```python
from build123d import *

# Parameters (mm, degrees)
SKETCH1_W           = 89.6
SKETCH1_H           = 100.6
BOSS_EXTRUDE1_DEPTH = 49.7
SKETCH4_W           = 16.6
SKETCH4_H           = 12
CUT_EXTRUDE1_DEPTH  = 120.117546986
SKETCH5_W           = 100.6
SKETCH5_H           = 3
BOSS_EXTRUDE2_DEPTH = 89.6
SKETCH7_R           = 4.175
BOSS_EXTRUDE3_DEPTH = 21.7
CUT_EXTRUDE2_START  = 21.7
SKETCH7_3_R         = 2.175
CUT_EXTRUDE2_DEPTH  = 5
SKETCH9_R           = 4.675
SKETCH9_R_2         = 2.175
BOSS_EXTRUDE4_DEPTH = 3.5
CUT_EXTRUDE4_START  = -1.5
SKETCH9_2_R         = 2.175
CUT_EXTRUDE4_DEPTH  = 1.5
SKETCH11_W          = 21.5
SKETCH11_H          = 17.55
SKETCH11_W_2        = 4.5
SKETCH11_H_2        = 7.5
BOSS_EXTRUDE5_DEPTH = 3.5
SKETCH12_W          = 17
SKETCH12_H          = 13.05
CUT_EXTRUDE5_DEPTH  = 3


with BuildPart() as part:
    # Sketch1 → Boss-Extrude1 (new body)
    with BuildSketch(Plane(origin=(0, 0, 0), x_dir=(1, 0, 0), z_dir=(0, 1, 0))):
        with BuildLine():
            Line((73.990371034, 53.1), (166.690371034, 53.1))
            ThreePointArc((166.690371034, 53.1), (169.518798158, 51.928427125), (170.690371034, 49.1))
            Line((170.690371034, 49.1), (170.690371034, -50.9))
            ThreePointArc((170.690371034, -50.9), (169.518798158, -53.728427125), (166.690371034, -54.9))
            Line((166.690371034, -54.9), (73.990371034, -54.9))
            Line((73.990371034, -54.9), (73.990371034, 53.1))
        make_face()
        with Locations((122.190371034, -0.9)):
            Rectangle(SKETCH1_W, SKETCH1_H, mode=Mode.SUBTRACT)
    extrude(amount=BOSS_EXTRUDE1_DEPTH)

    # Sketch4 → Cut-Extrude1 (cut, through all)
    with BuildSketch(Plane(origin=(77.390371034, 0, 0), x_dir=(0, 0, -1), z_dir=(1, 0, 0))):
        with Locations((37.1, 6)):
            Rectangle(SKETCH4_W, SKETCH4_H)
    extrude(amount=-CUT_EXTRUDE1_DEPTH, mode=Mode.SUBTRACT)

    # Sketch5 → Boss-Extrude2 (add)
    with BuildSketch(Plane(origin=(77.390371034, 0, 0), x_dir=(0, 0, -1), z_dir=(1, 0, 0))):
        with Locations((-0.9, 26.5)):
            Rectangle(SKETCH5_W, SKETCH5_H)
    extrude(amount=BOSS_EXTRUDE2_DEPTH)

    # Sketch7 → Boss-Extrude3 (add)
    with BuildSketch(Plane(origin=(0, 28, 0), x_dir=(1, 0, 0), z_dir=(0, 1, 0))):
        with Locations((78.928328283, 47.862042751)):
            Circle(SKETCH7_R)
        with Locations((165.452413785, 47.862042751)):
            Circle(SKETCH7_R)
        with Locations((165.452413785, -49.662042751)):
            Circle(SKETCH7_R)
        with Locations((78.928328283, -49.662042751)):
            Circle(SKETCH7_R)
    extrude(amount=BOSS_EXTRUDE3_DEPTH)

    # Sketch7<3> → Cut-Extrude2 (cut)
    with BuildSketch(Plane(origin=(0, 28, 0), x_dir=(1, 0, 0), z_dir=(0, 1, 0)).offset(CUT_EXTRUDE2_START)):
        with Locations(Location((78.928328283, 47.862042751, 0), (0, 0, 270))):
            Circle(SKETCH7_3_R)
        with Locations(Location((165.452413785, 47.862042751, 0), (0, 0, 270))):
            Circle(SKETCH7_3_R)
        with Locations(Location((165.452413785, -49.662042751, 0), (0, 0, 270))):
            Circle(SKETCH7_3_R)
        with Locations(Location((78.928328283, -49.662042751, 0), (0, 0, 270))):
            Circle(SKETCH7_3_R)
    extrude(amount=-CUT_EXTRUDE2_DEPTH, mode=Mode.SUBTRACT)

    # Sketch9 → Boss-Extrude4 (add)
    # profile 1 of 4: a face of its own
    with BuildSketch(Plane(origin=(0, 28, 0), x_dir=(1, 0, 0), z_dir=(0, 1, 0))):
        with Locations(Location((148.990371034, -14, 0), (0, 0, 90))):
            Circle(SKETCH9_R)
        with Locations(Location((148.990371034, -14, 0), (0, 0, 270))):
            Circle(SKETCH9_R_2, mode=Mode.SUBTRACT)
    # profile 2 of 4: a face of its own
    with BuildSketch(Plane(origin=(0, 28, 0), x_dir=(1, 0, 0), z_dir=(0, 1, 0))):
        with Locations(Location((99.990371034, -14, 0), (0, 0, 90))):
            Circle(SKETCH9_R)
        with Locations(Location((99.990371034, -14, 0), (0, 0, 270))):
            Circle(SKETCH9_R_2, mode=Mode.SUBTRACT)
    # profile 3 of 4: a face of its own
    with BuildSketch(Plane(origin=(0, 28, 0), x_dir=(1, 0, 0), z_dir=(0, 1, 0))):
        with Locations(Location((99.990371034, 27, 0), (0, 0, 90))):
            Circle(SKETCH9_R)
        with Locations(Location((99.990371034, 27, 0), (0, 0, 270))):
            Circle(SKETCH9_R_2, mode=Mode.SUBTRACT)
    # profile 4 of 4: a face of its own
    with BuildSketch(Plane(origin=(0, 28, 0), x_dir=(1, 0, 0), z_dir=(0, 1, 0))):
        with Locations(Location((148.990371034, 27, 0), (0, 0, 90))):
            Circle(SKETCH9_R)
        with Locations(Location((148.990371034, 27, 0), (0, 0, 270))):
            Circle(SKETCH9_R_2, mode=Mode.SUBTRACT)
    extrude(amount=BOSS_EXTRUDE4_DEPTH)

    # Sketch9<2> → Cut-Extrude4 (cut)
    with BuildSketch(Plane(origin=(0, 28, 0), x_dir=(1, 0, 0), z_dir=(0, 1, 0)).offset(CUT_EXTRUDE4_START)):
        with Locations(Location((99.990371034, 27, 0), (0, 0, 270))):
            Circle(SKETCH9_2_R)
        with Locations(Location((148.990371034, 27, 0), (0, 0, 270))):
            Circle(SKETCH9_2_R)
        with Locations(Location((99.990371034, -14, 0), (0, 0, 270))):
            Circle(SKETCH9_2_R)
        with Locations(Location((148.990371034, -14, 0), (0, 0, 270))):
            Circle(SKETCH9_2_R)
    extrude(amount=CUT_EXTRUDE4_DEPTH, mode=Mode.SUBTRACT)

    # Sketch11 → Boss-Extrude5 (add)
    with BuildSketch(Plane(origin=(0, 28, 0), x_dir=(1, 0, 0), z_dir=(0, 1, 0))):
        with Locations((131.240371034, -5.125)):
            Rectangle(SKETCH11_W, SKETCH11_H)
        with Locations((125.240371034, -7.65)):
            Rectangle(SKETCH11_W_2, SKETCH11_H_2, mode=Mode.SUBTRACT)
        with Locations((137.240371034, -2.6)):
            Rectangle(SKETCH11_W_2, SKETCH11_H_2, mode=Mode.SUBTRACT)
    extrude(amount=BOSS_EXTRUDE5_DEPTH)

    # Sketch12 → Cut-Extrude5 (cut)
    with BuildSketch(Plane.XZ.offset(-25)):
        with Locations((131.240371034, 5.125)):
            Rectangle(SKETCH12_W, SKETCH12_H)
    extrude(amount=-CUT_EXTRUDE5_DEPTH, mode=Mode.SUBTRACT)


solid = part.part
```
Could you check a few things on this model? Use its own coordinates, in mm. A direction names the side the tool comes from. Give positions to 0.01 mm unless a question says otherwise; leave off trailing zeros. Loops run counter-clockwise (first coordinate to the right, second up) from the corner with the lowest first, then second, coordinate; pieces in that order, holes last. Notation, with made-up numbers: (-22, -37) -> (4, -37) arc R9 cw to (4, -24) -> close; hole circle Ø8 at (-25, 84.5). An arc over 180 degrees is marked (long way). Put each result on its own line as item: value.
(1) Imagine slicing it at D-D on z = -27. Write out the boundary of the cut face in (x, y).
Computed:
outline: (73.99, 0) -> (77.39, 0) -> (77.39, 25) -> (166.99, 25) -> (166.99, 0) -> (170.69, 0) -> (170.69, 49.7) -> (166.99, 49.7) -> (166.99, 28) -> (153.67, 28) -> (153.67, 31.5) -> (151.17, 31.5) -> (151.17, 26.5) -> (146.82, 26.5) -> (146.82, 31.5) -> (144.32, 31.5) -> (144.32, 28) -> (104.67, 28) -> (104.67, 31.5) -> (102.17, 31.5) -> (102.17, 26.5) -> (97.82, 26.5) -> (97.82, 31.5) -> (95.32, 31.5) -> (95.32, 28) -> (77.39, 28) -> (77.39, 49.7) -> (73.99, 49.7) -> close
(2) Please list where these lines run through material, in increasing order: probe 1 along X at (y, z) = (27.65, -27); probe 2 along Z at (x, y) = (124, 29); probe 3 along X at (y, z) = (29, -27). Write a range as [from, to].
Computed:
probe 1: [73.99, 97.82], [102.17, 146.82], [151.17, 170.69]
probe 2: [-53.1, -49.4], [-3.65, 3.9], [11.4, 13.9], [51.2, 54.9]
probe 3: [73.99, 77.39], [95.32, 97.82], [102.17, 104.67], [144.32, 146.82], [151.17, 153.67], [166.99, 170.69]
(3) Thinking about a two-plate mould opening in X: for faces 1 (the face through (169.55, 24.502, 53.697)), 2 (the face through (131, 30, 13.9)), 3 (the face through (76, 49.7, -3)), which applies, pulls with the +X half, pulls with the -X half, needs draft (parallel to the pull), parting line crosses it, or undercut?
Computed:
face 1: pulls with the +X half
face 2: undercut
face 3: needs draft
(4) Imagine slicing it at C-C on y = 20. Write out the boundary of the cut face in (x, z).
Computed:
outline: (73.99, -53.1) -> (166.69, -53.1) arc R4 ccw to (170.69, -49.1) -> (170.69, 50.9) arc R4 ccw to (166.69, 54.9) -> (73.99, 54.9) -> close; hole (77.39, -49.4) -> (166.99, -49.4) -> (166.99, 51.2) -> (77.39, 51.2) -> close
(5) Imagine slicing it at B-B on x = 86. Write out the boundary of the cut face in (y, z), plus the area to 3 significant figures.
Computed:
outline: (0, -53.1) -> (49.7, -53.1) -> (49.7, -49.4) -> (28, -49.4) -> (28, 51.2) -> (49.7, 51.2) -> (49.7, 54.9) -> (0, 54.9) -> (0, 51.2) -> (25, 51.2) -> (25, -49.4) -> (0, -49.4) -> close
area: 670 mm^2
(6) I'm going to push flat-ended pins straight in: pin 1 Ø4 at (x, z) = (107.5, -35.5) entering from -Y; pin 2 Ø12 at (x, z) = (99, -40) entering from +Y; pin 3 Ø4 at (x, z) = (131.5, 5.5) entering from -Y. Where does each tip first touch, or does it pass through?
Computed:
pin 1: y = 25
pin 2: y = 28
pin 3: y = 28
(7) Imagine slicing it at A-A on y = 30. State how many separate pieces and enclosed holes the cut face has, plus the area to 3 significant figures.
Computed:
separate pieces: 6
enclosed holes: 7
area: 2,060 mm^2
(8) For faces 4 (the face through (76, 12, -37)), 5 (the face through (137, 30, -1.15)), 6 (the face through (122, 12, -49.4)), 7 (the face through (98.67, 28.96, -28.73)), which set-ups out of +Z, -Z, +X, -X, +Y, -Y let a thin tool reach every point of the face, with its end or its side?
Computed:
face 4: -X, -Y
face 5: +Y, -Y
face 6: -Y
face 7: +Y
